Source: CAD feature listing. Evaluate the final solid. Frame: model axes, mm. Face numbers are marked on the shaded views. A direction names the side the tool comes from. Give positions to 0.01 mm unless a question says otherwise; leave off trailing zeros. Order: outer loops, then holes, each group sorted by start corner. A loop starts at its lowest first (then second) coordinate and runs counter-clockwise, first axis right, second up.
1) Material intervals for line 1 (X direction, y = 1.5, z = -17) (3 decimals); line 2 (X direction, y = 7.5, z = -17) (3 decimals); line 3 (Z direction, x = -13.5, y = 5.75), sorted ascending.
2) Section C-C, the plane y = 3.25. Return loops of the section in (x, z) (3 decimals).
3) First-contact query: P1, Ø2, axis at y = 6, z = -22, coming from the -X side; P2, Ø1.5, axis at y = 1, z = -13, coming from the +X side; P3, Ø1.7, axis at x = -14.5, y = 5.5, coming from the +Z side; P4, Ø3, axis at x = -15.075, z = -17, coming from the +Y side. Flat tips, straight axial feed; report the tip coordinate or a pass-through.
4) Section B-B, the plane y = 8. Return loops of the section in (x, z) (3 decimals), plus the area to 3 significant figures.
5) Access query for the marked faces 1, 2, 3 and 4. Directions: +Z, -Z, +X, -X, +Y, -Y. A direction counts if a zero-diameter tool reaches every point of the face in a straight line with its end or side. Return the directions, or none.
6) Section A-A, the plane z = -17. Return loops of the section in (x, y) (3 decimals).
7) Draft query along X for the marked faces 5, 6 and 7. Return one class per face: released by +X, released by -X, zero draft, split by the parting line, or undercut.
Autodesk Inventor part; units mm, degrees
ref_plane "YZ Plane" through (0, 0, 0) normal (1, 0, 0) x (0, 1, 0)
ref_plane "XZ Plane" through (0, 0, 0) normal (0, 1, 0) x (-1, 0, 0)
ref_plane "XY Plane" through (0, 0, 0) normal (0, 0, 1) x (1, 0, 0)
sketch "Sketch1" plane through (0, 0, 0) normal (0, 1, 0) x (-1, 0, 0)
  line L0 (41.25, -2.25) -> (28.75, -2.25) construction
  line L1 (28.75, -2.25) -> (28.75, -14.75) construction
  line L2 (28.75, -14.75) -> (41.25, -14.75) construction
  line L3 (41.25, -14.75) -> (41.25, -2.25) construction
  line L4 (56.9183, -8.5) -> (8.3915, -8.5) construction
  line L5 (0, -17) -> (105, -17) construction
  line L6 (0, 0) -> (0, -51) construction
  line L7 (0, -34) -> (105, -34) construction
  line L8 (105, -51) -> (105, 0) construction
  line L9 (35, 19) -> (35, -51) construction
  line L10 (56.8064, -25.5) -> (17, -25.5) construction
  line L11 (28.75, -19.25) -> (28.75, -31.75) construction
  line L12 (41.25, -19.25) -> (28.75, -19.25) construction
  line L13 (41.25, -31.75) -> (41.25, -19.25) construction
  line L14 (28.75, -31.75) -> (41.25, -31.75) construction
  line L15 (28.75, -36.25) -> (28.75, -48.75) construction
  line L16 (41.25, -36.25) -> (28.75, -36.25) construction
  line L17 (41.25, -48.75) -> (41.25, -36.25) construction
  line L18 (28.75, -48.75) -> (41.25, -48.75) construction
  line L19 (56.3008, -42.5) -> (16.5498, -42.5) construction
  arc A0 (53.45, -12) -> (53.45, -22) centre (53.45, -17) ccw construction
  arc A1 (92, -22) -> (92, -12) centre (92, -17) ccw construction
  arc A2 (53.45, -29) -> (53.45, -39) centre (53.45, -34) ccw construction
  arc A3 (92, -39) -> (92, -29) centre (92, -34) ccw construction
  line L20 (53.45, -12) -> (92, -12) construction
  line L21 (53.45, -22) -> (92, -22) construction
  line L22 (53.45, -29) -> (92, -29) construction
  line L23 (53.45, -39) -> (92, -39) construction
  arc A4 (16.15, -38.8) -> (16.15, -29.2) centre (16.15, -34) ccw construction
  line L24 (103.5, -49.5) -> (103.5, -1.5) construction
  line L25 (1.5, -1.5) -> (1.5, -49.5) construction
  arc A5 (14, -29.2) -> (14, -38.8) centre (14, -34) ccw construction
  arc A6 (14, -12.2) -> (14, -21.8) centre (14, -17) ccw
  line L26 (16.15, -38.8) -> (14, -38.8) construction
  line L27 (14, -29.2) -> (16.15, -29.2) construction
  line L28 (14, -21.8) -> (16.15, -21.8)
  line L29 (16.15, -12.2) -> (14, -12.2)
  arc A7 (16.15, -21.8) -> (16.15, -12.2) centre (16.15, -17) ccw
  arc A8 (96.5, -51) -> (93, -47.5) centre (93, -51) ccw construction
  arc A9 (53.45, -47.5) -> (49.95, -51) centre (53.45, -51) ccw construction
  arc A10 (97.7697, -49.5) -> (93, -46) centre (93, -51) ccw construction
  line L30 (93, -46) -> (53.45, -46) construction
  line L31 (96.5, -51) -> (105, -51) construction
  line L32 (93, -47.5) -> (53.45, -47.5) construction
  line L33 (105, -49.5) -> (97.7697, -49.5) construction
  arc A11 (53.45, -46) -> (48.6803, -49.5) centre (53.45, -51) ccw construction
  arc A12 (48.6803, -1.5) -> (53.45, -5) centre (53.45, 0) ccw construction
  arc A13 (49.95, 0) -> (53.45, -3.5) centre (53.45, 0) ccw construction
  line L34 (93, -3.5) -> (53.45, -3.5) construction
  line L35 (93, -5) -> (53.45, -5) construction
  line L36 (97.7697, -1.5) -> (105, -1.5) construction
  line L37 (105, 0) -> (96.5, 0) construction
  arc A14 (93, -3.5) -> (96.5, 0) centre (93, 0) ccw construction
  arc A15 (93, -5) -> (97.7697, -1.5) centre (93, 0) ccw construction
  arc A16 (20.65, -51) -> (17.15, -47.5) centre (17.15, -51) ccw construction
  arc A17 (12, -47.5) -> (8.5, -51) centre (12, -51) ccw construction
  line L38 (17.15, -46) -> (12, -46) construction
  line L39 (17.15, -47.5) -> (12, -47.5) construction
  arc A18 (12, -46) -> (7.2303, -49.5) centre (12, -51) ccw construction
  arc A19 (21.9197, -49.5) -> (17.15, -46) centre (17.15, -51) ccw construction
  line L40 (48.6803, -49.5) -> (21.9197, -49.5) construction
  line L41 (7.2303, -49.5) -> (0, -49.5) construction
  line L42 (0, -51) -> (8.5, -51) construction
  line L43 (20.65, -51) -> (49.95, -51) construction
  line L44 (17.15, -5) -> (12, -5) construction
  line L45 (17.15, -3.5) -> (12, -3.5) construction
  arc A20 (8.5, 0) -> (12, -3.5) centre (12, 0) ccw construction
  arc A21 (17.15, -3.5) -> (20.65, 0) centre (17.15, 0) ccw construction
  arc A22 (7.2303, -1.5) -> (12, -5) centre (12, 0) ccw construction
  arc A23 (17.15, -5) -> (21.9197, -1.5) centre (17.15, 0) ccw construction
  line L46 (49.95, 0) -> (20.65, 0) construction
  line L47 (8.5, 0) -> (0, 0) construction
  line L48 (0, -1.5) -> (7.2303, -1.5) construction
  line L49 (21.9197, -1.5) -> (48.6803, -1.5) construction
  line L50 (113, 2) -> (-20, 2) construction
  line L51 (-20, 2) -> (-20, -53) construction
  line L52 (-20, -53) -> (113, -53) construction
  line L53 (113, -53) -> (113, 2) construction
  arc A24 (92, -23.5) -> (92, -10.5) centre (92, -17) ccw construction
  arc A25 (53.45, -10.5) -> (53.45, -23.5) centre (53.45, -17) ccw construction
  line L54 (92, -10.5) -> (53.45, -10.5) construction
  line L55 (53.45, -23.5) -> (92, -23.5) construction
  line L56 (15.075, -18.8909) -> (15.075, -15) construction
  arc A26 (16.15, -23.5) -> (16.15, -10.5) centre (16.15, -17) ccw
  arc A27 (14, -10.5) -> (14, -23.5) centre (14, -17) ccw
  line L57 (16.15, -23.5) -> (14, -23.5)
  line L58 (16.15, -10.5) -> (14, -10.5)
  point P0 (35, -8.5)
  point P1 (35, -42.5)
  point P2 (35, -25.5)
  point P3 (15.075, -17)
  dimension "d0" = 12.5
  dimension "d1" = 12.5
  dimension "d2" = 17
  dimension "d3" = 35
  dimension "d4" = 105
  dimension "d5" = 17
  dimension "d6" = 17
  dimension "d7" = 10
  dimension "d8" = 1.5
  dimension "d9" = 1.5
  dimension "d10" = 4.8
  dimension "d11" = 1.5
  dimension "d12" = 1.5
  dimension "d13" = 1.5
  dimension "d14" = 17
  dimension "d15" = 17
  dimension "d16" = 12
  dimension "d17" = 13
  dimension "d18" = 12.2
  dimension "d19" = 11.6
  dimension "d20" = 12.6
  dimension "d21" = 12
  dimension "d22" = 12.5
  dimension "d23" = 2
  dimension "d24" = 8
  dimension "d25" = 20
  dimension "d26" = 1.5
extrude "Extrusion3" add sketch "Sketch1" along normal blind 9.5 contours L29 A7 L28 A6
extrude "Extrusion4" add sketch "Sketch1" along normal blind 4
hole "Hole2" at (-35, 0, -8.5) at (0, 0, -17) at (-35, 0, -42.5) at (-35, 0, -25.5) at (-92, 0, -17) at (-53.45, 0, -17) at (-15.075, 0, -17) direction (0, 1, 0) diameter 4 end through all counterbore diameter 6 counterbore depth 3
chamfer "Chamfer2" distance 0.5 angle 45 4 edges at (-9.2, 9.5, -17) (-15.075, 9.5, -21.8) (-20.95, 9.5, -17) (-15.075, 9.5, -12.2)
properties part number "Small_retainer"
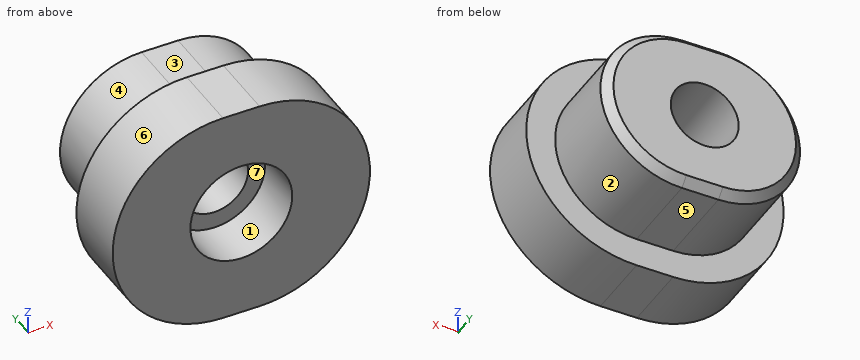
From the geometry:
1. line 1: x = -22.65 to -18.075, -12.075 to -7.5
1. line 2: x = -20.95 to -17.075, -13.075 to -9.2
1. line 3: z = -21.77 to -18.23, -15.77 to -12.23
2. outline: (-16.15, -23.5) - (-14, -23.5) arc R6.5 ccw to (-14, -10.5) - (-16.15, -10.5) arc R6.5 ccw to start; hole circle Ø4 at (-15.075, -17)
3. P1: stops at x = -18.8
3. P2: stops at x = -8.37
3. P3: stops at z = -12.2
3. P4: passes through
4. outline: (-16.15, -21.8) - (-14, -21.8) arc R4.8 ccw to (-14, -12.2) - (-16.15, -12.2) arc R4.8 ccw to start; hole circle Ø4 at (-15.075, -17)
4. area: 80.5 mm2
5. face 1: -Y
5. face 2: +X, +Y
5. face 3: +Z, +X, -X, +Y
5. face 4: -X, +Y
6. outline: (-22.65, 0) - (-18.075, 0) - (-18.075, 3) - (-17.075, 3) - (-17.075, 9.5) - (-20.45, 9.5) - (-20.95, 9) - (-20.95, 4) - (-22.65, 4) - close; (-13.075, 3) - (-12.075, 3) - (-12.075, 0) - (-7.5, 0) - (-7.5, 4) - (-9.2, 4) - (-9.2, 9) - (-9.7, 9.5) - (-13.075, 9.5) - close
7. face 5: zero draft
7. face 6: released by -X
7. face 7: undercut
